Check sheet for the modelled part. Datum: model origin and axes. Units: mm. A direction names the side the tool comes from. Coordinates: 2 decimals unless noted, no trailing zeros. Order: outer loops, then holes, each group sorted by start corner. A loop starts at its lowest first (then second) coordinate and runs counter-clockwise, first axis right, second up.
from build123d import *

# Parameters (mm, degrees)
SKETCH1_W           = 120
SKETCH1_H           = 40
BOSS_EXTRUDE1_DEPTH = 3
SKETCH2_W           = 3
SKETCH2_H           = 12.5
CUT_EXTRUDE1_DEPTH  = 64.316664473
SKETCH3_W           = 15
SKETCH3_H           = 3
CUT_EXTRUDE2_DEPTH  = 64.316664473


with BuildPart() as part:
    # Sketch1 → Boss-Extrude1 (new body)
    with BuildSketch(Plane(origin=(0, 0, 0), x_dir=(1, 0, 0), z_dir=(0, 1, 0))):
        Rectangle(SKETCH1_W, SKETCH1_H)
    extrude(amount=BOSS_EXTRUDE1_DEPTH)

    # Sketch2 → Cut-Extrude1 (cut, through all)
    with BuildSketch(Plane(origin=(0, 3, 0), x_dir=(1, 0, 0), z_dir=(0, 1, 0))):
        with Locations((-58.5, 13.75)):
            Rectangle(SKETCH2_W, SKETCH2_H)
        with Locations((-58.5, -13.75)):
            Rectangle(SKETCH2_W, SKETCH2_H)
        with Locations((58.5, 13.75)):
            Rectangle(SKETCH2_W, SKETCH2_H)
        with Locations((58.5, -13.75)):
            Rectangle(SKETCH2_W, SKETCH2_H)
    extrude(amount=-CUT_EXTRUDE1_DEPTH, mode=Mode.SUBTRACT)

    # Sketch3 → Cut-Extrude2 (cut, through all)
    with BuildSketch(Plane(origin=(0, 3, 0), x_dir=(1, 0, 0), z_dir=(0, 1, 0))):
        with Locations((-32.5, -18.5)):
            Rectangle(SKETCH3_W, SKETCH3_H)
        with Locations((32.5, -18.5)):
            Rectangle(SKETCH3_W, SKETCH3_H)
    extrude(amount=-CUT_EXTRUDE2_DEPTH, mode=Mode.SUBTRACT)


solid = part.part
(1) Go/stop test with flat-tipped pins: P1, Ø0.9, axis at x = 59, y = 2, coming from the -Z side; P2, Ø0.9, axis at y = 2, z = 12, coming from the +X side; P3, Ø1.5, axis at y = 1.5, z = -14.5, coming from the -X side. Record where each tip stops, or that it passes through.
Filled in:
P1: stops at z = -7.5
P2: stops at x = 57
P3: stops at x = -57
(2) Cross-section at B-B (z = -11). Enter the section's corners in (x, y).
Filled in:
outline: (-57, 0) - (57, 0) - (57, 3) - (-57, 3) - close
(3) Tool access check on faces 4 (the flat face through (-57, 2, -14)), 5 (the flat face through (-59, 2, 7.5)), 6 (the flat face through (0, 1, 20)), 7 (the flat face through (57, 2, -14)), 8 (the flat face through (25, 2, 19)). Record the directions out of +Z, -Z, +X, -X, +Y, -Y that give a thin tool (end or side, any length) a straight path to the whole face; none if there is none.
Filled in:
face 4: -Z, -X, +Y, -Y
face 5: +Z, -X, +Y, -Y
face 6: +Z, +X, -X, +Y, -Y
face 7: -Z, +X, +Y, -Y
face 8: +Z, +Y, -Y
(4) Thickness scan on probe 1 along X at (y, z) = (2, 18.5); probe 2 along X at (y, z) = (0.35, -12.5); probe 3 along Z at (x, y) = (-35.5, 2.65). Record the ranges inside material, lowest first.
Filled in:
probe 1: x = -57 to -40, -25 to 25, 40 to 57
probe 2: x = -57 to 57
probe 3: z = -20 to 17
(5) Cross-section at A-A (y = 0.55). Enter the section's corners in (x, z), and give its area (3 significant figures).
Filled in:
outline: (-60, -7.5) - (-57, -7.5) - (-57, -20) - (57, -20) - (57, -7.5) - (60, -7.5) - (60, 7.5) - (57, 7.5) - (57, 20) - (40, 20) - (40, 17) - (25, 17) - (25, 20) - (-25, 20) - (-25, 17) - (-40, 17) - (-40, 20) - (-57, 20) - (-57, 7.5) - (-60, 7.5) - close
area: 4,560 mm2
(6) Release check for a two-part mould opening along X. For faces 1 (the flat face through (57, 2, 14)), 2 (the flat face through (-59, 2, -7.5)), 3 (the flat face through (-33, 2, 17)) record: +X half, -X half, draft (parallel to the pull), parting line (faces both ways), or undercut.
Filled in:
face 1: +X half
face 2: draft
face 3: undercut
